The model under review builds one solid part; all positions refer to its coordinate system, in mm. A direction names the side the tool comes from. Give positions to 0.01 mm unless a question says otherwise; leave off trailing zeros. Loops run counter-clockwise (first coordinate to the right, second up) from the corner with the lowest first, then second, coordinate; pieces in that order, holes last. Notation, with made-up numbers: M 53,48 L 77,48 A34 cw 77,78 Z; hole C 68,-29.75 d6. An arc over 180 degrees is marked long. Put each result on its own line as item: value. Start each with the question number.
from build123d import *

# Parameters (mm, degrees)
SKETCH_1_W               = 20
SKETCH_1_H               = 15
EXTRUDE_1_DEPTH          = 30
EXTRUDE_2_DEPTH          = 6
EXTRUDE_2_DEPTH_BACK     = 6
SKETCH_3_R               = 1.35
EXTRUDE_3_DEPTH          = 11.5
EXTRUDE_START            = -0.2
EXTRUDE_4_DEPTH          = 29.6
EXTRUDE_5_DEPTH          = 14.6
FILLET_1_R               = 0.1
FILLET_2_R               = 0.2
SKETCH_6_R               = 1.25
CUT_EXTRUDE_1_DEPTH      = 38.165171868
SKETCH_7_R               = 1.25
CUT_EXTRUDE_2_DEPTH      = 40.449334595
SKETCH_8_R               = 1.25
CUT_EXTRUDE_3_DEPTH      = 5
CUT_EXTRUDE_4_DEPTH      = 5
CUT_EXTRUDE_4_DEPTH_BACK = 5
FILLET_3_R               = 0.1


with BuildPart() as part:
    # 草图1 → 凸台-拉伸1 (new body)
    with BuildSketch(Plane.XY):
        Rectangle(SKETCH_1_W, SKETCH_1_H)
    extrude(amount=-EXTRUDE_1_DEPTH)

    # 草图2 → 凸台-拉伸2 (add, two sides: drawn at the far end of the back side and taken through both)
    with BuildSketch(Plane(origin=(0, 0, 0), x_dir=(1, 0, 0), z_dir=(0, 1, 0)).offset(-EXTRUDE_2_DEPTH_BACK)):
        with BuildLine():
            Line((-4.25, 0), (-5.75, 0))
            Line((-5.75, 0), (-5.75, -0.638562172))
            ThreePointArc((-5.75, -0.638562172), (-5, -2.3), (-4.25, -0.638562172))
            Line((-4.25, -0.638562172), (-4.25, 0))
        make_face()
        with BuildLine():
            Line((4.25, 0), (4.25, -0.638562172))
            ThreePointArc((4.25, -0.638562172), (5, -2.3), (5.75, -0.638562172))
            Line((5.75, -0.638562172), (5.75, 0))
            Line((5.75, 0), (4.25, 0))
        make_face()
    extrude(amount=EXTRUDE_2_DEPTH + EXTRUDE_2_DEPTH_BACK)

    # 草图3 → 凸台-拉伸3 (add)
    with BuildSketch(Plane.XY):
        with Locations(Location((0, 0, 0), (0, 0, 180))):
            Circle(SKETCH_3_R)
    extrude(amount=EXTRUDE_3_DEPTH)

    # 草图4 → 凸台-拉伸4 (add)
    with BuildSketch(Plane.XY.offset(EXTRUDE_START)):
        with BuildLine():
            Line((-1.5, 7.5), (-1.5, 8.177124344))
            ThreePointArc((-1.5, 8.177124344), (-1.780042303, 8.588161527), (-1.95, 9.055590279))
            Line((-1.95, 9.055590279), (-1.95, 10))
            Line((-1.95, 10), (-1.165769145, 10))
            Line((-1.165769145, 10), (-0.5, 8.57225346))
            Line((-0.5, 8.57225346), (-0.5, 7.5))
            Line((-0.5, 7.5), (-1.5, 7.5))
        make_face()
        with BuildLine():
            Line((1.5, 7.5), (1.5, 8.177124344))
            ThreePointArc((1.5, 8.177124344), (1.780042303, 8.588161527), (1.95, 9.055590279))
            Line((1.95, 9.055590279), (1.95, 10))
            Line((1.95, 10), (1.165769145, 10))
            Line((1.165769145, 10), (0.5, 8.57225346))
            Line((0.5, 8.57225346), (0.5, 7.5))
            Line((0.5, 7.5), (1.5, 7.5))
        make_face()
    extrude(amount=-EXTRUDE_4_DEPTH)

    # 草图5 → 凸台-拉伸5 (add)
    with BuildSketch(Plane(origin=(0, 7.5, 0), x_dir=(-1, 0, 0), z_dir=(0, 1, 0)).offset(EXTRUDE_START)):
        with BuildLine():
            Line((1.5, -30), (1.5, -30.677124344))
            ThreePointArc((1.5, -30.677124344), (1.780042303, -31.088161527), (1.95, -31.555590279))
            Line((1.95, -31.555590279), (1.95, -32.5))
            Line((1.95, -32.5), (1.165769145, -32.5))
            Line((1.165769145, -32.5), (-1.165769145, -32.5))
            Line((-1.165769145, -32.5), (-1.95, -32.5))
            Line((-1.95, -32.5), (-1.95, -31.555590279))
            ThreePointArc((-1.95, -31.555590279), (-1.780042303, -31.088161527), (-1.5, -30.677124344))
            Line((-1.5, -30.677124344), (-1.5, -30))
            Line((-1.5, -30), (-0.5, -30))
            Line((-0.5, -30), (0.5, -30))
            Line((0.5, -30), (1.5, -30))
        make_face()
    extrude(amount=-EXTRUDE_5_DEPTH)

    # 圆角1
    fillet_1_edges = [part.edges().sort_by_distance(p)[0] for p in [
        (-1.557884573, 10, -29.8),
        (-1.95, 10, -15),
        (-1.165769145, 10, -15),
        (-1.557884573, 10, -0.2),
        (1.557884573, 10, -29.8),
        (1.165769145, 10, -15),
        (1.95, 10, -15),
        (1.557884573, 10, -0.2),
        (1.95, 0, -32.5),
        (0, -7.3, -32.5),
        (-1.95, 0, -32.5),
        (0, 7.3, -32.5),
    ]]
    fillet(fillet_1_edges, radius=FILLET_1_R)

    # 圆角2
    fillet_2_edges = [part.edges().sort_by_distance(p)[0] for p in [
        (10, 0, -30),
        (0, 7.5, -30),
        (-10, 0, -30),
        (0, 7.5, 0),
        (10, 0, 0),
        (0, -7.5, 0),
        (-10, 0, 0),
        (0, -7.5, -30),
        (-10, 7.5, -15),
        (10, 7.5, -15),
        (10, -7.5, -15),
        (-10, -7.5, -15),
    ]]
    fillet(fillet_2_edges, radius=FILLET_2_R - 0.0001)  # a hair under: the kernel refuses the full size

    # 草图6 → 切除-拉伸1 (cut, through all)
    with BuildSketch(Plane(origin=(0, 7.5, 0), x_dir=(-1, 0, 0), z_dir=(0, 1, 0))):
        with Locations(Location((7.5, -27.5, 0), (0, 0, 90))):
            Circle(SKETCH_6_R)
        with Locations(Location((-7.5, -27.5, 0), (0, 0, 90))):
            Circle(SKETCH_6_R)
    extrude(amount=-CUT_EXTRUDE_1_DEPTH, mode=Mode.SUBTRACT)

    # 草图7 → 切除-拉伸2 (cut, through all)
    with BuildSketch(Plane.ZY.offset(10)):
        with Locations((-27.5, -5)):
            Circle(SKETCH_7_R)
    extrude(amount=-CUT_EXTRUDE_2_DEPTH, mode=Mode.SUBTRACT)

    # 草图8 → 切除-拉伸3 (cut)
    with BuildSketch(Plane(origin=(0, 0, -30), x_dir=(-1, 0, 0), z_dir=(0, 0, -1))):
        with Locations((-7.5, 0)):
            Circle(SKETCH_8_R)
        with Locations((7.5, 0)):
            Circle(SKETCH_8_R)
    extrude(amount=-CUT_EXTRUDE_3_DEPTH, mode=Mode.SUBTRACT)

    # 草图9 → 切除-拉伸4 (cut, two sides: drawn at the far end of the back side and taken through both)
    with BuildSketch(Plane(origin=(0, 0, 0), x_dir=(0, 0, -1), z_dir=(1, 0, 0)).offset(-CUT_EXTRUDE_4_DEPTH_BACK)):
        with BuildLine():
            Line((32.5, 1.95), (31.555590279, 1.95))
            ThreePointArc((31.555590279, 1.95), (31.088161527, 1.780042303), (30.677124344, 1.5))
            Line((30.677124344, 1.5), (30, 1.5))
            Line((30, 1.5), (30, 7.95))
            Line((30, 7.95), (32.5, 7.95))
            Line((32.5, 7.95), (32.5, 1.95))
        make_face()
        with BuildLine():
            Line((30, -1.5), (30.677124344, -1.5))
            ThreePointArc((30.677124344, -1.5), (31.088161527, -1.780042303), (31.555590279, -1.95))
            Line((31.555590279, -1.95), (32.5, -1.95))
            Line((32.5, -1.95), (32.5, -7.95))
            Line((32.5, -7.95), (30, -7.95))
            Line((30, -7.95), (30, -1.5))
        make_face()
    extrude(amount=CUT_EXTRUDE_4_DEPTH + CUT_EXTRUDE_4_DEPTH_BACK, mode=Mode.SUBTRACT)

    # 圆角3
    fillet_3_edges = [part.edges().sort_by_distance(p)[0] for p in [
        (1.95, 1.95, -31.97779514),
        (1.920710678, 1.95, -32.470710678),
        (-1.95, 1.95, -31.97779514),
        (-1.920710678, 1.95, -32.470710678),
        (1.95, -1.95, -31.97779514),
        (1.920710678, -1.95, -32.470710678),
        (-1.95, -1.95, -31.97779514),
        (-1.920710678, -1.95, -32.470710678),
        (0, 1.95, -32.5),
        (0, -1.95, -32.5),
    ]]
    fillet(fillet_3_edges, radius=FILLET_3_R)


solid = part.part
(1) We need section B-B, the plane z = 1.3. Write out the cut boundary in (x, y).
(2) We need section C-C, the plane y = 3. Write out the cut boundary in (x, z).
(3) Insertion check: pin 1 (1 mm diameter, centred on x = -6.5, y = -1.5, fed in from -Z); pin 2 (0.7 mm diameter, centred on y = -0.5, z = -32, fed in from -X); pin 3 (12 mm diameter, centred on x = 2, z = -20.5, fed in from +Y); pin 4 (0.6 mm diameter, centred on x = 5, z = 1.5, fed in from +Y). Each pin has a flat end and moves straight along its axis. Give the tip position at first contact, or say it passes through.
(4) To check wall thickness, follow L1, parallel to X at y = 0, z = -26.9; L2, parallel to Z at x = -7.5, y = -2.2; L3, parallel to Z at x = 0.5, y = 2.5. State the ranges of each line that lie inside material, in increasing order. Write a range as [from, to].
(5) We need section A-A, the plane x = 0. Write out the cut boundary in (y, z).
(6) For faces 4 (the flat face through (-1.95, 0, -32)), 5 (the cylindrical face through (1.777, 8.582, -14.793)), 6 (the cylindrical face through (-6.579, 0.845, -29.045)), 7 (the cylindrical face through (-1.777, 0.027, -31.082)), 8 (the flat face through (-0.824, 9.267, -14.793)), list the 3-axis set-ups (+Z, -Z, +X, -X, +Y, -Y) from which the entire face can be reached by the end or side of a thin tool; tool diameter is ignored.
(7) We need section D-D, the plane y = -5.5. Write out the cut boundary in (x, z), plus the area to 3 significant figures.
(8) Draft analysis for pull direction Z (two halves, no side actions). For faces 1 (the cylindrical face through (5, -0.1, 2.3)), 2 (the flat face through (0, 1.95, -32)), 3 (the flat face through (0, 0, -32.5)), state which applies: +Z half, -Z half, draft (parallel to the pull), parting line (faces both ways), or undercut.
Check sheet entries:
1. outline: M -6,-6 L -4,-6 L -4,6 L -6,6 Z; C 0,0 d2.7; M 4,-6 L 6,-6 L 6,6 L 4,6 Z
2. outline: M -10,-29.8 A0.2 ccw -9.8,-30 L 9.8,-30 A0.2 ccw 10,-29.8 L 10,-0.2 A0.2 ccw 9.8,0 L 5.75,0 L 5.75,0.64 A1 ccw long 4.25,0.64 L 4.25,0 L -4.25,0 L -4.25,0.64 A1 ccw long -5.75,0.64 L -5.75,0 L -9.8,0 A0.2 ccw -10,-0.2 Z; hole C -7.5,-27.5 d2.5; hole C 7.5,-27.5 d2.5
3. pin 1: stops at z = -30
3. pin 2: stops at x = -1.95
3. pin 3: stops at y = 10
3. pin 4: stops at y = 6
4. L1: x = [-10, -8.75], [-6.25, 6.25], [8.75, 10]
4. L2: z = [-30, -28.75], [-26.25, 0]
4. L3: z = [-30, 0]
5. outline: M -7.5,-29.8 A0.2 ccw -7.3,-30 L -1.5,-30 L -1.5,-30.68 A2 ccw -1.95,-31.56 L -1.95,-32.4 A0.1 ccw -1.85,-32.5 L 1.85,-32.5 A0.1 ccw 1.95,-32.4 L 1.95,-31.56 A2 ccw 1.5,-30.68 L 1.5,-30 L 7.3,-30 A0.2 ccw 7.5,-29.8 L 7.5,-0.2 A0.2 ccw 7.3,0 L 1.35,0 L 1.35,11.5 L -1.35,11.5 L -1.35,0 L -7.3,0 A0.2 ccw -7.5,-0.2 Z; hole C -5,-27.5 d2.5
6. face 4: -Z, -X, +Y, -Y
6. face 5: +Z, -Z, +X
6. face 6: -Z
6. face 7: -X, +Y, -Y
6. face 8: +Z, -Z, +Y
7. outline: M -10,-29.8 A0.2 ccw -9.8,-30 L 9.8,-30 A0.2 ccw 10,-29.8 L 10,-28.65 L 8,-28.65 A1.25 cw 7,-28.65 L -7,-28.65 A1.25 cw -8,-28.65 L -10,-28.65 Z; M -10,-26.35 L -8,-26.35 A1.25 cw -7,-26.35 L 7,-26.35 A1.25 cw 8,-26.35 L 10,-26.35 L 10,-0.2 A0.2 ccw 9.8,0 L 5.75,0 L 5.75,0.64 A1 ccw long 4.25,0.64 L 4.25,0 L -4.25,0 L -4.25,0.64 A1 ccw long -5.75,0.64 L -5.75,0 L -9.8,0 A0.2 ccw -10,-0.2 Z
7. area: 561 mm²
8. face 1: undercut
8. face 2: draft
8. face 3: -Z half
